Autodesk Inventor part; units mm, degrees
ref_plane "YZ Plane" through (0, 0, 0) normal (1, 0, 0) x (0, 1, 0)
ref_plane "XZ Plane" through (0, 0, 0) normal (0, 1, 0) x (-1, 0, 0)
ref_plane "XY Plane" through (0, 0, 0) normal (0, 0, 1) x (1, 0, 0)
sketch "Sketch1" plane through (0, 0, 0) normal (0, 0, 1) x (1, 0, 0)
  line L0 (-0.515, 0.509) -> (-4.515, 0.509)
  line L1 (-4.515, -14.491) -> (-0.515, -14.491)
  line L2 (-0.515, -14.491) -> (-0.515, 0.509)
  line L3 (-4.515, -1.991) -> (-4.126, -1.991)
  line L4 (-4.126, -1.991) -> (-4.126, -4.981)
  line L5 (-4.126, -4.981) -> (-4.515, -4.981)
  line L6 (-4.515, -4.981) -> (-4.515, -1.991)
  line L7 (-4.515, -8.981) -> (-4.126, -8.981)
  line L8 (-4.126, -8.981) -> (-4.126, -11.991)
  line L9 (-4.126, -11.991) -> (-4.515, -11.991)
  line L10 (-4.515, -11.991) -> (-4.515, -8.981)
  line L11 (-4.515, 0.509) -> (-4.515, -1.991)
  line L12 (-4.515, -4.981) -> (-4.515, -14.491)
  point P0 (0, 0)
  dimension "d0" = 4
  dimension "d1" = 15
  dimension "d2" = 0.389
  dimension "d3" = 2.99
  dimension "d4" = 4
  dimension "d5" = 2.5
  dimension "d6" = 3.01
extrude "Extrusion1" add sketch "Sketch1" along normal blind 10 contours L2 L1 L12 L9 L8 L7 L5 L4 L3 L11 L0
sketch "Sketch6" plane through (0, 0, 10) normal (0, 0, 1) x (1, 0, 0)
  line L0 (-0.515, 0.509) -> (-0.515, -14.491)
  line L1 (-0.515, -0.4166) -> (-1.3203, -0.1235)
  line L2 (-1.3203, -0.1235) -> (-1.3203, 0.0462)
  line L3 (-1.3203, 0.2159) -> (-0.515, 0.509)
  line L4 (-1.3203, 0.2159) -> (-1.3203, 0.0462)
  line L5 (-0.515, 0.509) -> (-0.515, -0.4166)
  line L6 (-0.412, -0.4191) -> (-1.6665, -0.4191) construction
  line L7 (-1.3203, -1.0542) -> (-0.515, -1.3473)
  line L8 (-0.515, -1.3473) -> (-0.515, -0.4216)
  line L9 (-1.3203, -1.0542) -> (-1.3203, -0.8845)
  line L10 (-1.3203, -0.7148) -> (-1.3203, -0.8845)
  line L11 (-0.515, -0.4216) -> (-1.3203, -0.7148)
  line L12 (-0.1629, -1.3498) -> (-1.5742, -1.3498) construction
  line L13 (-1.3203, -2.9154) -> (-0.515, -3.2085)
  line L14 (-0.515, -3.2085) -> (-0.515, -2.2829)
  line L15 (-1.3203, -2.9154) -> (-1.3203, -2.7457)
  line L16 (-1.3203, -2.576) -> (-1.3203, -2.7457)
  line L17 (-0.515, -2.2829) -> (-1.3203, -2.576)
  line L18 (-1.3203, -1.6454) -> (-0.515, -1.3523)
  line L19 (-0.515, -1.3523) -> (-0.515, -2.2779)
  line L20 (-1.3203, -1.6454) -> (-1.3203, -1.8151)
  line L21 (-1.3203, -1.9848) -> (-1.3203, -1.8151)
  line L22 (-0.515, -2.2779) -> (-1.3203, -1.9848)
  line L23 (-0.071, -3.211) -> (-1.4404, -3.211) construction
  line L24 (-1.3203, -6.6379) -> (-0.515, -6.9311)
  line L25 (-0.515, -6.9311) -> (-0.515, -6.0054)
  line L26 (-1.3203, -6.6379) -> (-1.3203, -6.4682)
  line L27 (-1.3203, -6.2985) -> (-1.3203, -6.4682)
  line L28 (-0.515, -6.0054) -> (-1.3203, -6.2985)
  line L29 (-1.3203, -5.3679) -> (-0.515, -5.0748)
  line L30 (-0.515, -5.0748) -> (-0.515, -6.0004)
  line L31 (-1.3203, -5.3679) -> (-1.3203, -5.5376)
  line L32 (-1.3203, -5.7073) -> (-1.3203, -5.5376)
  line L33 (-0.515, -6.0004) -> (-1.3203, -5.7073)
  line L34 (-1.3203, -3.5067) -> (-0.515, -3.2135)
  line L35 (-0.515, -3.2135) -> (-0.515, -4.1392)
  line L36 (-1.3203, -3.5067) -> (-1.3203, -3.6764)
  line L37 (-1.3203, -3.846) -> (-1.3203, -3.6764)
  line L38 (-0.515, -4.1392) -> (-1.3203, -3.846)
  line L39 (-0.515, -4.1442) -> (-1.3203, -4.4373)
  line L40 (-0.515, -5.0698) -> (-0.515, -4.1442)
  line L41 (-1.3203, -4.7767) -> (-0.515, -5.0698)
  line L42 (-1.3203, -4.7767) -> (-1.3203, -4.607)
  line L43 (-1.3203, -4.4373) -> (-1.3203, -4.607)
  line L44 (0.2425, -6.9336) -> (-1.3203, -6.9336) construction
  line L45 (-1.3203, -8.4992) -> (-0.515, -8.7923)
  line L46 (-0.515, -8.7923) -> (-0.515, -7.8667)
  line L47 (-0.515, -7.8667) -> (-1.3203, -8.1598)
  line L48 (-1.3203, -8.1598) -> (-1.3203, -8.3295)
  line L49 (-1.3203, -8.4992) -> (-1.3203, -8.3295)
  line L50 (-1.3203, -7.2292) -> (-0.515, -6.9361)
  line L51 (-1.3203, -7.2292) -> (-1.3203, -7.3989)
  line L52 (-1.3203, -7.5686) -> (-1.3203, -7.3989)
  line L53 (-0.515, -7.8617) -> (-1.3203, -7.5686)
  line L54 (-0.515, -6.9361) -> (-0.515, -7.8617)
  line L55 (-1.3203, -10.9517) -> (-0.515, -10.6586)
  line L56 (-0.515, -10.6586) -> (-0.515, -11.5842)
  line L57 (-1.3203, -10.9517) -> (-1.3203, -11.1214)
  line L58 (-1.3203, -11.2911) -> (-1.3203, -11.1214)
  line L59 (-0.515, -11.5842) -> (-1.3203, -11.2911)
  line L60 (-0.515, -9.7279) -> (-1.3203, -10.0211)
  line L61 (-1.3203, -10.0211) -> (-1.3203, -10.1908)
  line L62 (-1.3203, -10.3605) -> (-1.3203, -10.1908)
  line L63 (-1.3203, -10.3605) -> (-0.515, -10.6536)
  line L64 (-0.515, -10.6536) -> (-0.515, -9.7279)
  line L65 (-0.515, -8.7973) -> (-0.515, -9.7229)
  line L66 (-0.515, -9.7229) -> (-1.3203, -9.4298)
  line L67 (-1.3203, -9.0904) -> (-1.3203, -9.2601)
  line L68 (-1.3203, -9.4298) -> (-1.3203, -9.2601)
  line L69 (-1.3203, -9.0904) -> (-0.515, -8.7973)
  line L70 (-4.515, -8.981) -> (-4.515, -4.981)
  line L71 (0.0056, -11.5867) -> (-1.782, -11.5867) construction
  line L72 (-1.3203, -16.5355) -> (-0.515, -16.2424)
  line L73 (-1.3203, -16.5355) -> (-1.3203, -16.7052)
  line L74 (-1.3203, -16.8749) -> (-1.3203, -16.7052)
  line L75 (-0.515, -17.168) -> (-1.3203, -16.8749)
  line L76 (-0.515, -16.2424) -> (-0.515, -17.168)
  line L77 (-0.515, -15.3117) -> (-1.3203, -15.6048)
  line L78 (-1.3203, -15.6048) -> (-1.3203, -15.7745)
  line L79 (-1.3203, -15.9442) -> (-0.515, -16.2374)
  line L80 (-1.3203, -15.9442) -> (-1.3203, -15.7745)
  line L81 (-0.515, -16.2374) -> (-0.515, -15.3117)
  line L82 (-0.515, -14.3811) -> (-0.515, -15.3067)
  line L83 (-0.515, -15.3067) -> (-1.3203, -15.0136)
  line L84 (-1.3203, -15.0136) -> (-1.3203, -14.8439)
  line L85 (-1.3203, -14.6742) -> (-1.3203, -14.8439)
  line L86 (-1.3203, -14.6742) -> (-0.515, -14.3811)
  line L87 (-1.3203, -14.083) -> (-0.515, -14.3761)
  line L88 (-1.3203, -14.083) -> (-1.3203, -13.9133)
  line L89 (-1.3203, -13.7436) -> (-1.3203, -13.9133)
  line L90 (-0.515, -13.4505) -> (-1.3203, -13.7436)
  line L91 (-0.515, -14.3761) -> (-0.515, -13.4505)
  line L92 (-0.515, -13.4455) -> (-1.3203, -13.1524)
  line L93 (-1.3203, -13.1524) -> (-1.3203, -12.9827)
  line L94 (-1.3203, -12.813) -> (-1.3203, -12.9827)
  line L95 (-1.3203, -12.813) -> (-0.515, -12.5198)
  line L96 (-0.515, -12.5198) -> (-0.515, -13.4455)
  line L97 (-1.3203, -12.2217) -> (-0.515, -12.5148)
  line L98 (-1.3203, -12.2217) -> (-1.3203, -12.052)
  line L99 (-1.3203, -11.8823) -> (-1.3203, -12.052)
  line L100 (-0.515, -11.5892) -> (-1.3203, -11.8823)
  line L101 (-0.515, -12.5148) -> (-0.515, -11.5892)
  dimension "d70" = 0
  dimension "d71" = 0
  dimension "d72" = 70
  dimension "d73" = 0.8053
  dimension "d74" = 70
  dimension "d76" = 0.1697
  dimension "d77" = 110
  dimension "d78" = 70
  dimension "d79" = 40
  dimension "d80" = 0.9256
  dimension "d81" = 0.0025
  dimension "d82" = 0.0025
  dimension "d83" = 0.0025
  dimension "d84" = 0.0025
  dimension "d87" = 0.0025
extrude "Extrusion4" cut sketch "Sketch6" against normal through all contours L0 L82 L83 L84 L85 L86 | L0 L87 L88 L89 L90 | L0 L92 L93 L94 L95 | L0 L97 L98 L99 L100 | L0 L59 L58 L57 L55 | L0 L63 L62 L61 L60 | L0 L66 L68 L67 L69 | L0 L45 L49 L48 L47 | L0 L53 L52 L51 L50 | L0 L24 L26 L27 L28 | L0 L33 L32 L31 L29 | L0 L41 L42 L43 L39 | L0 L38 L37 L36 L34 | L0 L13 L15 L16 L17 | L0 L22 L21 L20 L18 | L0 L7 L9 L10 L11 | L0 L1 L2 L4 L3
equation "\"d14\" = 15.81278"
equation "\"d15\" = 20deg"
equation "\"d16\" = 8.01181"
equation "\"d17\" = 10.54185"
equation "\"d18\" = 3.31182"
equation "\"d24\" = 15.81278"
equation "\"d25\" = 20deg"
equation "\"d26\" = 8.01181"
equation "\"d27\" = 10.54185"
equation "\"d28\" = 3.31182"
equation "\"d35\" = 15.81278"
equation "\"d36\" = 20deg"
equation "\"d37\" = 8.01181"
equation "\"d38\" = 10.54185"
equation "\"d39\" = 3.31182"
equation "\"d59\" = 3.35558"
equation "\"d60\" = 20deg"
equation "\"d61\" = 2.55024"
equation "\"d62\" = 3.35558"
equation "\"d63\" = 1.05419"
properties part number "rack2"
The model under review builds one solid part; all positions refer to its coordinate system, in mm. A direction names the side the tool comes from. Round coordinates to 2 decimals unless told otherwise and drop trailing zeros. Order: outer loops, then holes, each group sorted by start corner. A loop starts at its lowest first (then second) coordinate and runs counter-clockwise, first axis right, second up. Notation, with made-up numbers: (49, -12.75) -> (65, -12.75) arc R16 cw to (65, -8.75) -> close; hole circle Ø5 at (24.5, 16). An arc over 180 degrees is marked (long way). Use CSV: the item, a comma, the result in double quotes. Start each with the question number.
(1) Mouldability with a two-part tool opening along Y and no side actions: class faces 1 (the face through (-0.91, -9.58, 5.07)), 2 (the face through (-4.515, -1, 5)) as pulls with the +Y half, pulls with the -Y half, needs draft (parallel to the pull), parting line crosses it, or undercut.
(2) Consider section A-A on y = -9.25. Write out the cut boundary in (x, z), and give its area (3 significant figures).
(3) Wall thickness on probe 1 along Y at (x, z) = (-4.2, 5); probe 2 along X at (y, z) = (-7.5, 1) (3 decimals): over which ranges is each line inside the solid? List them lowest first. Write a range as from..to.
(4) Tool access review of faces 3 (the face through (-0.92, -3.06, 5.07)), 4 (the face through (-4.515, -13, 5)): name each direction out of +Z, -Z, +X, -X, +Y, -Y from which nothing blocks a thin tool from reaching the whole face with its end or side.
(5) Insertion check: pin 1 (3.5 mm diameter, centred on y = -3.5, z = 2.5, fed in from -X) (3 decimals); pin 2 (2.5 mm diameter, centred on y = -10.5, z = 7, fed in from -X). Each pin has a flat end and moves straight along its axis. Give the tip position at first contact, or say it passes through.
Responses:
1,face 1,"undercut"
1,face 2,"needs draft"
2,outline,"(-4.13, 0) -> (-1.32, 0) -> (-1.32, 10) -> (-4.13, 10) -> close"
2,area,"28.1 mm²"
3,probe 1,"-14.49..-11.99, -8.98..-4.98, -1.99..0.51"
3,probe 2,"-4.515..-1.32"
4,face 3,"+Z, -Z, +X"
4,face 4,"+Z, -Z, -X, +Y, -Y"
5,pin 1,"x = -4.515"
5,pin 2,"x = -4.13"
